The model under review builds one solid part; all positions refer to its coordinate system, in mm. A direction names the side the tool comes from. Coordinates: 2 decimals unless noted, no trailing zeros. Loops run counter-clockwise (first coordinate to the right, second up) from the corner with the lowest first, then second, coordinate; pieces in that order, holes last. Notation, with made-up numbers: (17, 61.25) - (23, 61.25) arc R22 ccw to (23, 99.25) - close; hole circle Ø11 at (22.25, 88.5). An arc over 180 degrees is marked (long way). One line per item, written item: value. Start each with the question number.
1. We need section A-A, the plane y = 27.1. Give the boundary of the cut face in (x, z).
2. Insertion check: P1, Ø7, axis at x = 76, z = 8.5, coming from the -Y side; P2, Ø1, axis at y = 21, z = 7, coming from the +X side; P3, Ø1.5, axis at y = 16, z = 6.5, coming from the -X side; P4, Ø2, axis at x = 45.1, y = 11.1, coming from the -Z side. Each pin has a flat end and moves straight along its axis. Give the tip position at first contact, or say it passes through.
3. To check wall thickness, follow line 1 (Y direction, x = 79, z = 8.25); line 2 (Y direction, x = 45.1, z = 1.3); line 3 (X direction, y = 49, z = 3.25). State the ranges of each line that lie inside material, in increasing order.
4. We need section B-B, the plane x = 81.1. Give the boundary of the cut face in (y, z), then the cut area to 3 significant figures.
5. We need section D-D, the plane x = 65.1. Give the boundary of the cut face in (y, z).
6. For faces 5 (the face through (56, 52.2, 8)), 6 (the face through (107.2, 26.8, 15)), 7 (the face through (56.366, 27.409, 7.463)), list the 3-axis set-ups (+Z, -Z, +X, -X, +Y, -Y) from which the entire face can be reached by the end or side of a thin tool; tool diameter is ignored.
7. Mouldability with a two-part tool opening along Y and no side actions: class faces 1 (the face through (106.61, 3.56, 14.97)), 2 (the face through (2, 27, 8)), 3 (the face through (5, 27, 10)), 4 (the face through (106.64, 50.61, 14.97)) as +Y half, -Y half, draft (parallel to the pull), parting line (faces both ways), or undercut.
8. We need section C-C, the plane z = 6. Give the boundary of the cut face in (x, y), then the cut area to 3 significant figures.
from build123d import *

# Parameters (mm, degrees)
F1_DEPTH = 3
F2_W     = 100.2
F2_H     = 44.2
F3_DEPTH = 14
F4_SIZE2 = 4
F4_SIZE  = 2
F5_R     = 19.5
F5_R_2   = 1.75
F6_DEPTH = 3.001
F7_W     = 3
F7_H     = 44.2
F8_DEPTH = 10
F8_TAPER = 3
F9_R     = 1


with BuildPart() as f1:
    # F0 (on Top) → F1 (new body)
    with BuildSketch(Plane.XY):
        with BuildLine():
            ThreePointArc((0, 5), (1.4644660941, 1.4644660941), (5, 0))
            Line((5, 0), (105.2, 0))
            ThreePointArc((105.2, 0), (108.7355339059, 1.4644660941), (110.2, 5))
            Line((110.2, 5), (110.2, 49.2))
            ThreePointArc((110.2, 49.2), (108.7355339059, 52.7355339059), (105.2, 54.2))
            Line((105.2, 54.2), (5, 54.2))
            ThreePointArc((5, 54.2), (1.4644660941, 52.7355339059), (0, 49.2))
            Line((0, 49.2), (0, 5))
        make_face()
    extrude(amount=F1_DEPTH)

    # F2 (on face) → F3 (join)
    with BuildSketch(Plane.XY.offset(3)):
        with BuildLine():
            ThreePointArc((2, 5), (2.8786796564, 2.8786796564), (5, 2))
            Line((5, 2), (105.2, 2))
            ThreePointArc((105.2, 2), (107.3213203436, 2.8786796564), (108.2, 5))
            Line((108.2, 5), (108.2, 49.2))
            ThreePointArc((108.2, 49.2), (107.3213203436, 51.3213203436), (105.2, 52.2))
            Line((105.2, 52.2), (5, 52.2))
            ThreePointArc((5, 52.2), (2.8786796564, 51.3213203436), (2, 49.2))
            Line((2, 49.2), (2, 5))
        make_face()
        with Locations((55.1, 27.1)):
            Rectangle(F2_W, F2_H, mode=Mode.SUBTRACT)
    extrude(amount=F3_DEPTH)

    # F4
    f4_edges = [f1.edges().sort_by_distance(p)[0] for p in [
        (55.1, 2, 17),
    ]]
    f4_side = f1.faces().sort_by_distance((3.709296, 3.709296, 17))[0]
    chamfer(f4_edges, length=F4_SIZE, length2=F4_SIZE2, reference=f4_side)

    # F5 (on face) → F6 (cut, through all)
    with BuildSketch(Plane.XY.offset(3)):
        with Locations((29.1, 27.1)):
            Circle(F5_R)
        with Locations((13.1, 43.1)):
            Circle(F5_R_2)
        with Locations((13.1, 11.1)):
            Circle(F5_R_2)
        with Locations((45.1, 11.1)):
            Circle(F5_R_2)
        with Locations((45.1, 43.1)):
            Circle(F5_R_2)
        with Locations((81.1, 27.1)):
            Circle(F5_R)
        with Locations((65.1, 43.1)):
            Circle(F5_R_2)
        with Locations((65.1, 11.1)):
            Circle(F5_R_2)
        with Locations((97.1, 11.1)):
            Circle(F5_R_2)
        with Locations((97.1, 43.1)):
            Circle(F5_R_2)
    extrude(amount=-F6_DEPTH, mode=Mode.SUBTRACT)

    # F7 (on face) → F8 (join)
    with BuildSketch(Plane.XY.offset(3)):
        with Locations((55.1, 27.1)):
            Rectangle(F7_W, F7_H)
    extrude(amount=F8_DEPTH, taper=F8_TAPER)

    # F9
    f9_edges = [f1.edges().sort_by_distance(p)[0] for p in [
        (56.075922, 27.1, 13),
        (54.124078, 27.1, 13),
    ]]
    fillet(f9_edges, radius=F9_R)


solid = f1.part
Findings below:
1. outline: (0, 0) - (9.6, 0) - (9.6, 3) - (5, 3) - (5, 17) - (4, 17) - (2, 13) - (2, 3) - (0, 3) - close; (48.6, 0) - (61.6, 0) - (61.6, 3) - (56.6, 3) - (56.13, 12.05) arc R1 ccw to (55.13, 13) - (55.07, 13) arc R1 ccw to (54.07, 12.05) - (53.6, 3) - (48.6, 3) - close; (100.6, 0) - (110.2, 0) - (110.2, 3) - (108.2, 3) - (108.2, 13) - (106.2, 17) - (105.2, 17) - (105.2, 3) - (100.6, 3) - close
2. P1: y = 2
2. P2: x = 108.2
2. P3: x = 2
2. P4: through
3. line 1: 2 to 5, 49.2 to 52.2
3. line 2: 0 to 9.35, 12.85 to 15.95, 38.25 to 41.35, 44.85 to 54.2
3. line 3: 2 to 5, 53.61 to 56.59, 105.2 to 108.2
4. outline: (0, 0) - (7.6, 0) - (7.6, 3) - (5, 3) - (5, 17) - (4, 17) - (2, 13) - (2, 3) - (0, 3) - close; (46.6, 0) - (54.2, 0) - (54.2, 3) - (52.2, 3) - (52.2, 13) - (50.2, 17) - (49.2, 17) - (49.2, 3) - (46.6, 3) - close
4. area: 122 mm2
5. outline: (0, 0) - (9.35, 0) - (9.35, 3) - (5, 3) - (5, 17) - (4, 17) - (2, 13) - (2, 3) - (0, 3) - close; (12.85, 0) - (15.95, 0) - (15.95, 3) - (12.85, 3) - close; (38.25, 0) - (41.35, 0) - (41.35, 3) - (38.25, 3) - close; (44.85, 0) - (54.2, 0) - (54.2, 3) - (52.2, 3) - (52.2, 13) - (50.2, 17) - (49.2, 17) - (49.2, 3) - (44.85, 3) - close
6. face 5: +Z, +X, -X, +Y
6. face 6: +Z, +X, +Y, -Y
6. face 7: +Z
7. face 1: -Y half
7. face 2: draft
7. face 3: undercut
7. face 4: +Y half
8. outline: (2, 5) arc R3 ccw to (5, 2) - (105.2, 2) arc R3 ccw to (108.2, 5) - (108.2, 49.2) arc R3 ccw to (105.2, 52.2) - (5, 52.2) arc R3 ccw to (2, 49.2) - close; (53.76, 5.16) - (56.44, 5.16) - (56.44, 49.04) - (53.76, 49.04) - close; hole (5, 5) - (105.2, 5) - (105.2, 49.2) - (5, 49.2) - close
8. area: 1,010 mm2
